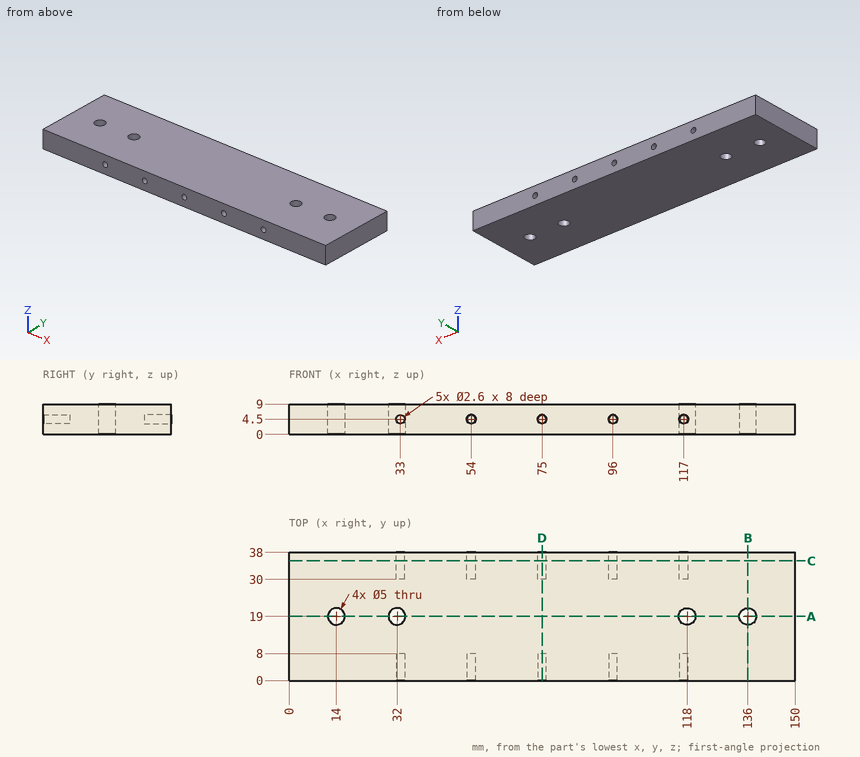
Design review of the part shown in the three views and the two pictorial views. Dimensions are in mm from the part's minimum x, y and z. Coordinates: 2 decimals unless noted, no trailing zeros. Loops run counter-clockwise (first coordinate to the right, second up) from the corner with the lowest first, then second, coordinate; pieces in that order, holes last. Notation, with made-up numbers: M -16,-7 L 34,-7 A17 ccw 34,13 Z; hole C 30.5,84 d5. An arc over 180 degrees is marked long. Put each result on its own line as item: value. Start each with the question number.
Q1. Clearance check with flat-ended pins moving along their axes: pin 1 (0.8 mm diameter, centred on x = 54.5, z = 4, fed in from +Y); pin 2 (0.8 mm diameter, centred on x = 74.5, z = 4.5, fed in from -Y). State where each tip first meets the part, or that it passes through.
Q2. Add section D-D (x = 75). Write out the cut boundary in (y, z).
Q3. Add section A-A (y = 19). Write out the cut boundary in (x, z), and give its area (3 significant figures).
Q4. Add section C-C (y = 35.5). Write out the cut boundary in (x, z).
Q5. Add section B-B (x = 136). Write out the cut boundary in (y, z), and give its area (3 significant figures).
Q6. Wall thickness on line 1 (X direction, y = 32.75, z = 4.5); line 2 (Y direction, x = 14, z = 7); line 3 (Z direction, x = 96, y = 5): over which ranges is each line inside the solid? List them lowest first.
Answers:
1. pin 1: stops at y = 30
1. pin 2: stops at y = 8
2. outline: M 0,0 L 38,0 L 38,3.2 L 30,3.2 L 30,5.8 L 38,5.8 L 38,9 L 0,9 L 0,5.8 L 8,5.8 L 8,3.2 L 0,3.2 Z
3. outline: M 0,0 L 11.5,0 L 11.5,9 L 0,9 Z; M 16.5,0 L 29.5,0 L 29.5,9 L 16.5,9 Z; M 34.5,0 L 115.5,0 L 115.5,9 L 34.5,9 Z; M 120.5,0 L 133.5,0 L 133.5,9 L 120.5,9 Z; M 138.5,0 L 150,0 L 150,9 L 138.5,9 Z
3. area: 1,170 mm^2
4. outline: M 0,0 L 150,0 L 150,9 L 0,9 Z; hole C 33,4.5 d2.6; hole C 54,4.5 d2.6; hole C 75,4.5 d2.6; hole C 96,4.5 d2.6; hole C 117,4.5 d2.6
5. outline: M 0,0 L 16.5,0 L 16.5,9 L 0,9 Z; M 21.5,0 L 38,0 L 38,9 L 21.5,9 Z
5. area: 297 mm^2
6. line 1: x = 0 to 31.7, 34.3 to 52.7, 55.3 to 73.7, 76.3 to 94.7, 97.3 to 115.7, 118.3 to 150
6. line 2: y = 0 to 16.5, 21.5 to 38
6. line 3: z = 0 to 3.2, 5.8 to 9
